from build123d import *

# Parameters (mm, degrees)
BOSS_EXTRUDE1_DEPTH                   = 35.56
FILLET1_R                             = 12.7
F_7_8_0_875_DIAMETER_HOLE1_D          = 22.225
SKETCH6_W                             = 24.384
SKETCH6_H                             = 44.958
CUT_EXTRUDE1_DEPTH                    = 2.794
FILLET2_R                             = 1.27
F_40_0_098_DIAMETER_HOLE1_D           = 2.4892
F_40_0_098_DIAMETER_HOLE1_CSINK_D     = 3.7592
F_40_0_098_DIAMETER_HOLE1_CSINK_ANGLE = 90
CUT_EXTRUDE3_DEPTH                    = 63.260576162
CUT_EXTRUDE4_DEPTH                    = 63.260576162


with BuildPart() as part:
    # Sketch1 → Boss-Extrude1 (new body)
    with BuildSketch(Plane.XY):
        Polygon((0, 0), (0, 50.8), (-5.588, 50.8), (-5.588, 17.78), (-1.916643762, 0), align=None)
    extrude(amount=BOSS_EXTRUDE1_DEPTH)

    # Fillet1
    fillet1_edges = [part.edges().sort_by_distance(p)[0] for p in [
        (-5.588, 17.78, 17.78),
    ]]
    fillet(fillet1_edges, radius=FILLET1_R)

    # 7/8 (0.875) Diameter Hole1 (through all)
    with Locations(Plane.ZY.offset(5.588)):
        with Locations((17.415519888, 39.229457165)):
            Hole(F_7_8_0_875_DIAMETER_HOLE1_D / 2)

    # Sketch6 → Cut-Extrude1 (cut)
    with BuildSketch(Plane(origin=(0, 0, 0), x_dir=(0, 0, -1), z_dir=(1, 0, 0))):
        with Locations((-17.580042727, 28.321)):
            Rectangle(SKETCH6_W, SKETCH6_H)
    extrude(amount=-CUT_EXTRUDE1_DEPTH, mode=Mode.SUBTRACT)

    # Fillet2
    fillet2_edges = [part.edges().sort_by_distance(p)[0] for p in [
        (-1.397, 5.842, 29.772042727),
        (-1.397, 5.842, 5.388042727),
    ]]
    fillet(fillet2_edges, radius=FILLET2_R)

    # #40 (0.098) Diameter Hole1 (through all)
    with Locations(Plane.ZY.offset(5.588)):
        with Locations((32.415519888, 43.729457165), (32.652313364, 26.212120957), (32.415519888, 9.729457165), (25.915519888, 3.429457165), (8.915519888, 3.429457165), (2.642788208, 9.215688736), (2.415519888, 26.729457165), (2.415519888, 43.729457165)):
            CounterSinkHole(F_40_0_098_DIAMETER_HOLE1_D / 2, F_40_0_098_DIAMETER_HOLE1_CSINK_D / 2, counter_sink_angle=F_40_0_098_DIAMETER_HOLE1_CSINK_ANGLE)

    # Sketch10 → Cut-Extrude3 (cut, through all)
    with BuildSketch(Plane(origin=(0, 0, 0), x_dir=(0, 0, -1), z_dir=(1, 0, 0))):
        Polygon((-35.56, 44.780420684), (-30.397580851, 50.8), (-35.56, 50.8), align=None)
    extrude(amount=-CUT_EXTRUDE3_DEPTH, mode=Mode.SUBTRACT)

    # Sketch11 → Cut-Extrude4 (cut, through all)
    with BuildSketch(Plane(origin=(0, 0, 0), x_dir=(0, 0, -1), z_dir=(1, 0, 0))):
        Polygon((-5.085545117, 50.8), (0, 50.8), (0, 44.824895363), align=None)
        Polygon((0, 6.029531172), (-5.128692816, 0), (0, 0), align=None)
        Polygon((-35.56, 6.07121688), (-35.56, 0), (-30.417091858, 0), align=None)
    extrude(amount=-CUT_EXTRUDE4_DEPTH, mode=Mode.SUBTRACT)


solid = part.part
Could you check a few things on this model? Use its own coordinates, in mm. A direction names the side the tool comes from. Coordinates: 2 decimals unless noted, no trailing zeros. Order: outer loops, then holes, each group sorted by start corner. A loop starts at its lowest first (then second) coordinate and runs counter-clockwise, first axis right, second up. Notation, with made-up numbers: (12, -24.75) - (38, -24.75) arc R20 cw to (38, -16.75) - close; hole circle Ø6 at (13, -18.5). An arc over 180 degrees is marked (long way). Answer in a Markdown table with one row per item. Add a question column.
(1) If we section it at C-C, the plane x = -0.85: State how many separate pieces and enclosed holes the cut face has, then the cut area to 3 significant figures.
(2) I need wall thicknesses on L1, parallel to Z at x = -0.8, y = 18.5; L2, parallel to Y at x = -1.6, z = 3; L3, parallel to Z at x = -0.3, y = 6. Which ranges of each line are inside material? Lowest first, please.
(3) If we mould it in two halves opening along Y, with no side actions, what happens to faces 1 (the face through (-2.442, 27.963, 2.578)), 2 (the face through (-2.44, 44.78, 1.75)), 3 (the face through (-1, 5.842, 18)), 4 (the face through (0, 20, 5))? For each: released by +Y, released by -Y, zero draft, split by the parting line, or undercut.
(4) Will these pins go through, and if not, where does the flat tip stop? pin 1 (2 mm diameter, centred on x = -1, y = 37, fed in from -Z); pin 2 (1 mm diameter, centred on x = -2.5, z = 31.5, fed in from -Y); pin 3 (5 mm diameter, centred on y = 24, z = 22.5, fed in from +X); pin 4 (0.8 mm diameter, centred on x = -2, z = 16, fed in from +Y).
(5) If we section it at A-A, the plane y = 38.5: Please give me the cut outline in (x, z).
(6) If we section it at B-B, the plane z = 8.5: Please give me the cut outline in (x, y).
(7) If we section it at D-D, the plane z = 23.5: Please give me the cut outline in (x, y).
(8) On a 3-axis mill with a long thin cutter (end or side, diameter ignored), from which of +Z, -Z, +X, -X, +Y, -Y can I reach the whole of each face in a straight line? I mean faces 5 (the face through (-1, 29, 29.772)), 6 (the face through (-5.588, 28, 14)). Say none if no direction works.
Results are:
| question | item | result |
|---|---|---|
| 1 | separate pieces | 1 |
| 1 | enclosed holes | 8 |
| 1 | area | 610 mm2 |
| 2 | L1 | z = 0 to 5.39, 29.77 to 35.56 |
| 2 | L2 | y = 2.5 to 8.02, 10.41 to 25.63, 27.83 to 42.63, 44.83 to 48.35 |
| 2 | L3 | z = 0.03 to 6.04, 29.12 to 35.5 |
| 3 | face 1 | undercut |
| 3 | face 2 | undercut |
| 3 | face 3 | released by +Y |
| 3 | face 4 | zero draft |
| 4 | pin 1 | stops at z = 0 |
| 4 | pin 2 | stops at y = 0.92 |
| 4 | pin 3 | stops at x = -2.79 |
| 4 | pin 4 | stops at y = 5.84 |
| 5 | outline | (-5.59, 0) - (0, 0) - (0, 5.39) - (-2.79, 5.39) - (-2.79, 6.33) - (-5.59, 6.33) - close; (-5.59, 28.5) - (-2.79, 28.5) - (-2.79, 29.77) - (0, 29.77) - (0, 35.56) - (-5.59, 35.56) - close |
| 6 | outline | (-5.59, 19.08) arc R12.7 ccw to (-5.33, 16.51) - (-2.87, 4.6) - (0, 4.6) - (0, 5.84) - (-2.79, 5.84) - (-2.79, 32.6) - (-5.59, 32.6) - close; (-5.59, 45.86) - (-2.79, 45.86) - (-2.79, 50.8) - (-5.59, 50.8) - close; (-2.38, 2.26) - (-1.92, 0) - (0, 0) - (0, 2.26) - close |
| 7 | outline | (-5.59, 19.08) arc R12.7 ccw to (-5.33, 16.51) - (-1.92, 0) - (0, 0) - (0, 5.84) - (-2.79, 5.84) - (-2.79, 29.93) - (-5.59, 29.93) - close; (-5.59, 48.53) - (-2.79, 48.53) - (-2.79, 50.8) - (-5.59, 50.8) - close |
| 8 | face 5 | +X, +Y |
| 8 | face 6 | +Z, -Z, -X, +Y, -Y |
